Work out the finished part from the listing and answer in its coordinate system (mm). Face numbers are marked on the shaded views. A direction names the side the tool comes from. Round coordinates to 2 decimals unless told otherwise and drop trailing zeros. Loops run counter-clockwise (first coordinate to the right, second up) from the corner with the lowest first, then second, coordinate; pieces in that order, holes last. Notation, with made-up numbers: (29.25, 88) -> (70.25, 88) arc R5 ccw to (70.25, 97) -> close; hole circle Ø9 at (60, 28). An arc over 180 degrees is marked (long way). Use one line per item in the form item = value.
```python
from build123d import *

# Parameters (mm, degrees)
SKETCH1_W           = 76.2
SKETCH1_H           = 31.75
BOSS_EXTRUDE1_DEPTH = 31.75
SHELL4_T            = 2.54
CUT_EXTRUDE5_START  = 34.29
SKETCH2_R           = 11.811
CUT_EXTRUDE5_DEPTH  = 12.7
FILLET3_R           = 2.54


with BuildPart() as part:
    # Sketch1 → Boss-Extrude1 (new body)
    with BuildSketch(Plane(origin=(0, 0, 0), x_dir=(1, 0, 0), z_dir=(0, 1, 0))):
        with Locations((9.130718954, 1.390359477)):
            Rectangle(SKETCH1_W, SKETCH1_H)
    extrude(amount=BOSS_EXTRUDE1_DEPTH)

    # Shell4
    shell4_openings = [part.faces().sort_by_distance(p)[0] for p in [
        (9.130718954, 0, -1.390359477),
    ]]
    offset(amount=SHELL4_T, openings=shell4_openings, kind=Kind.INTERSECTION)

    # Sketch2 → Cut-Extrude5 (cut, symmetric)
    with BuildSketch(Plane(origin=(0, 0, 0), x_dir=(1, 0, 0), z_dir=(0, 1, 0)).offset(CUT_EXTRUDE5_START)):
        with Locations(Location((9.130718954, 1.390359477, 0), (0, 0, 270))):
            Circle(SKETCH2_R)
    extrude(amount=CUT_EXTRUDE5_DEPTH, both=True, mode=Mode.SUBTRACT)

    # Fillet3
    fillet3_edges = [part.edges().sort_by_distance(p)[0] for p in [
        (49.770718954, 34.29, -1.390359477),
        (9.130718954, 34.29, -19.805359477),
        (9.130718954, 34.29, -13.201359477),
        (-31.509281046, 34.29, -1.390359477),
        (-31.509281046, 17.145, -19.805359477),
        (49.770718954, 17.145, -19.805359477),
    ]]
    fillet(fillet3_edges, radius=FILLET3_R - 0.0001)  # a hair under: the kernel refuses the full size


solid = part.part
```
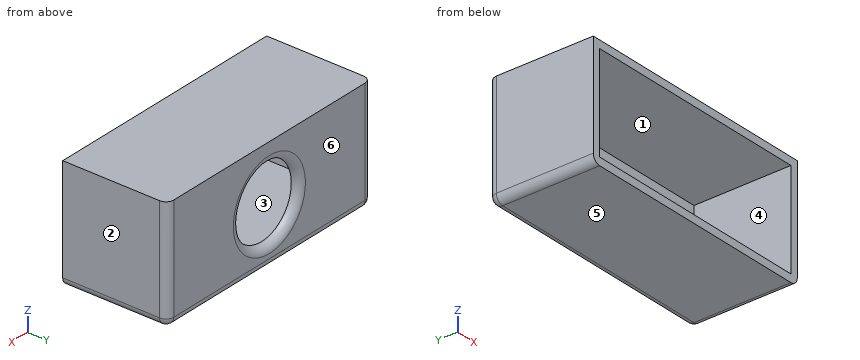
(1) For a pull along Z with two mould halves and no side action, classify the marked faces 3, 4, 5 and 6 as +Z half, -Z half, draft (parallel to the pull), parting line (faces both ways), or undercut.
Completed:
face_3 = undercut
face_4 = undercut
face_5 = -Z half
face_6 = draft
(2) Find section B-B, the plane x = 35. Write down the section's boundary in (y, z), then the cut area to 3 significant figures.
Completed:
outline = (0, -19.81) -> (31.75, -19.81) arc R2.54 ccw to (34.29, -17.27) -> (34.29, 17.02) -> (0, 17.02) -> (0, 14.48) -> (31.75, 14.48) -> (31.75, -17.27) -> (0, -17.27) -> close
area = 253 mm2
(3) Find section A-A, the plane y = 30. Write down the section's boundary in (x, z).
Completed:
outline = (-31.51, -17.27) arc R2.54 ccw to (-28.97, -19.81) -> (47.23, -19.81) arc R2.54 ccw to (49.77, -17.27) -> (49.77, 17.02) -> (-31.51, 17.02) -> close; hole (-28.97, -17.27) -> (47.23, -17.27) -> (47.23, 14.48) -> (-28.97, 14.48) -> close
(4) Consider L1, parallel to Z at x = -3.5, y = 24; L2, parallel to X at y = 21, z = -1; L3, parallel to Y at x = -16, z = -1. Determine where each line is inside the solid, lowest interval first.
Completed:
L1 = -19.81 to -17.27, 14.48 to 17.02
L2 = -31.51 to -28.97, 47.23 to 49.77
L3 = 31.75 to 34.29
(5) For the marked faces 1 and 2, determine the directions among +Z, -Z, +X, -X, +Y, -Y from which every point of the face is accessible in a straight line to the end or side of a thin tool.
Completed:
face_1 = -Y
face_2 = +Z, -Z, +X, +Y, -Y
